Part print with two shaded views. Sizes in mm from the minimum x, y, z corner. Round coordinates to 2 decimals unless told otherwise and drop trailing zeros. Write each loop counter-clockwise with the first axis right and the second up, starting at its lowest first coordinate (ties: lowest second). Pieces come first, ordered by that corner, then holes.
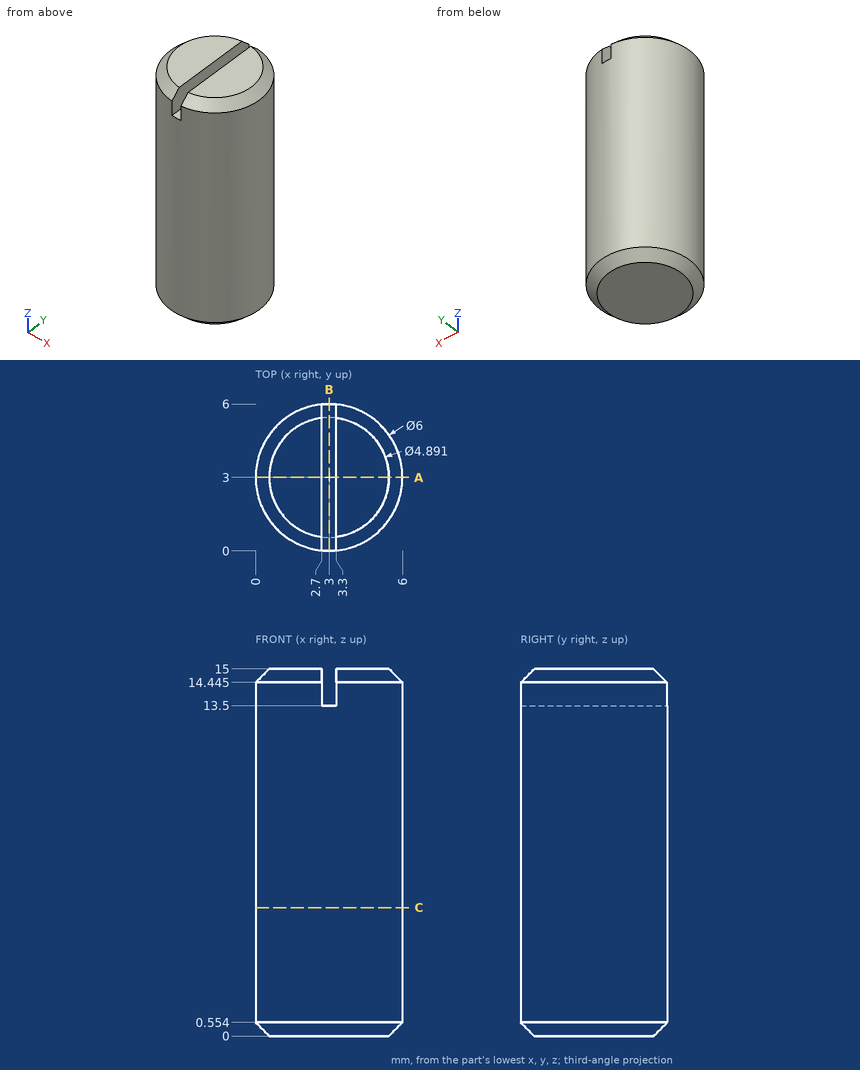
Q1. Wall check: L1, parallel to Y at x = 3.1, z = 9.75; L2, parallel to X at y = 2.15, z = 0.5; L3, parallel to Y at x = 0.4, z = 4 (1 decimal). Give the ranges that are in metal, low to high.
Values follow:
L1: y = 0 to 6
L2: x = 0.18 to 5.82
L3: y = 1.5 to 4.5
Q2. Cut at B-B on x = 3. Write the cut outline in (y, z) (1 decimal), plus the area to 3 significant figures.
Values follow:
outline: (0, 0.6) - (0.6, 0) - (5.4, 0) - (6, 0.6) - (6, 13.5) - (0, 13.5) - close
area: 80.7 mm2
Q3. Cut at A-A on y = 3. Write the cut outline in (x, z) (1 decimal).
Values follow:
outline: (0, 0.6) - (0.6, 0) - (5.4, 0) - (6, 0.6) - (6, 14.4) - (5.4, 15) - (3.3, 15) - (3.3, 13.5) - (2.7, 13.5) - (2.7, 15) - (0.6, 15) - (0, 14.4) - close
Q4. Cut at C-C on z = 5.25. Write the cut outline in (x, y).
Values follow:
outline: circle Ø6 at (3, 3)
